The model under review builds one solid part; all positions refer to its coordinate system, in mm. Face numbers are marked on the shaded views. A direction names the side the tool comes from. Round coordinates to 2 decimals unless told otherwise and drop trailing zeros. Write each loop counter-clockwise with the first axis right and the second up, starting at its lowest first coordinate (ties: lowest second). Pieces come first, ordered by that corner, then holes. Notation, with made-up numbers: (60.5, 54) -> (89.5, 54) arc R19 ccw to (89.5, 64) -> close; hole circle Ø4 at (-28.5, 1.5). An arc over 180 degrees is marked (long way). Use CSV: the item, a comma, the result in double quotes. Start each with the question number.
1) Take a section at A-A, the plane x = 22.5. Give the boundary of the cut face in (y, z).
2) Machinability: for the marked faces 1, 2, 3 and 4, which of the approach directions +Z, -Z, +X, -X, +Y, -Y give a long, thin tool a straight path to every point of the face, cutting with its end or side? Answer none if there is none.
3) Take a section at C-C, the plane y = -6.75. Give the boundary of the cut face in (x, z).
4) Mouldability with a two-part tool opening along X and no side actions: class the marked faces 5, 6, 7 and 8 as released by +X, released by -X, zero draft, split by the parting line, or undercut.
5) Wall thickness on probe 1 along X at (y, z) = (9.75, 4.25); probe 2 along Y at (x, z) = (0, 8.25); probe 3 along Y at (x, z) = (4.5, 5.5): over which ranges is each line inside the solid? List them lowest first. Write a range as [from, to].
6) For pin 1 Ø8 at (x, y) = (27.5, 11.5) entering from +Z; pin 2 Ø3 at (y, z) = (8, 5.5) entering from +X; pin 3 Ø5 at (x, z) = (28, 3.5) entering from +Y; pin 4 Ø5 at (x, z) = (25, 7) entering from -Y, all flat-tipped, find the tip position at first contact; note any pin that passes through.
7) Take a section at B-B, the plane z = 2.5. State how many separate pieces and enclosed holes the cut face has, then the cut area to 3 significant figures.
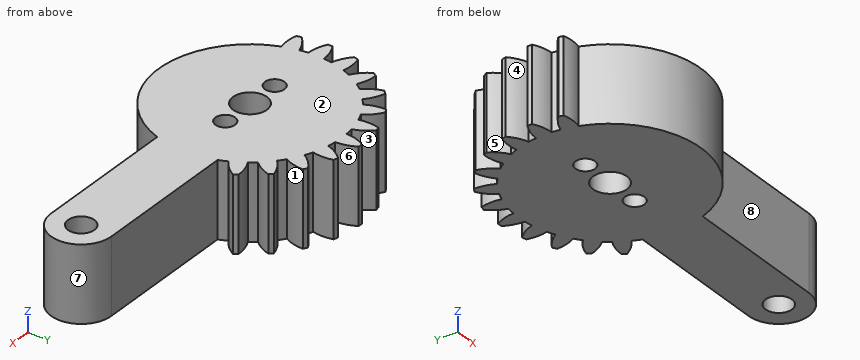
from build123d import *

# Parameters (mm, degrees)
SKETCH1_R           = 1.75
BOSS_EXTRUDE1_DEPTH = 10
SKETCH2_R           = 1.3
SKETCH2_R_2         = 2.25
CUT_EXTRUDE1_DEPTH  = 40.007683858


with BuildPart() as part:
    # Sketch1 → Boss-Extrude1 (new body)
    with BuildSketch(Plane.XY):
        with BuildLine():
            Line((0.31, 14.63), (-0.31, 14.63))
            ThreePointArc((-0.31, 14.63), (-0.838273314, 13.383704325), (-1.04, 12.04518576))
            ThreePointArc((-1.04, 12.04518576), (-1.578061664, 11.986568374), (-2.112960617, 11.903927815))
            ThreePointArc((-2.112960617, 11.903927815), (-2.65424773, 13.144626757), (-3.487085624, 14.211728743))
            Line((-3.487085624, 14.211728743), (-4.085959636, 14.051260935))
            ThreePointArc((-4.085959636, 14.051260935), (-4.273667417, 12.71070456), (-4.122086336, 11.365584201))
            ThreePointArc((-4.122086336, 11.365584201), (-4.626642697, 11.169703548), (-5.12192646, 10.951436862))
            ThreePointArc((-5.12192646, 10.951436862), (-5.965886177, 12.009764599), (-7.046532125, 12.824951657))
            Line((-7.046532125, 12.824951657), (-7.583467875, 12.514951657))
            ThreePointArc((-7.583467875, 12.514951657), (-7.417818147, 11.171491285), (-6.9232593, 9.911436862))
            ThreePointArc((-6.9232593, 9.911436862), (-7.359925677, 9.591641884), (-7.781841479, 9.252623584))
            ThreePointArc((-7.781841479, 9.252623584), (-8.870959341, 10.05645683), (-10.125769107, 10.564175311))
            Line((-10.125769107, 10.564175311), (-10.564175311, 10.125769107))
            ThreePointArc((-10.564175311, 10.125769107), (-10.05645683, 8.870959341), (-9.252623584, 7.781841479))
            ThreePointArc((-9.252623584, 7.781841479), (-9.591641884, 7.359925677), (-9.911436862, 6.9232593))
            ThreePointArc((-9.911436862, 6.9232593), (-11.171491285, 7.417818147), (-12.514951657, 7.583467875))
            Line((-12.514951657, 7.583467875), (-12.824951657, 7.046532125))
            ThreePointArc((-12.824951657, 7.046532125), (-12.009764599, 5.965886177), (-10.951436862, 5.12192646))
            ThreePointArc((-10.951436862, 5.12192646), (-11.169703548, 4.626642697), (-11.365584201, 4.122086336))
            ThreePointArc((-11.365584201, 4.122086336), (-12.71070456, 4.273667417), (-14.051260935, 4.085959636))
            Line((-14.051260935, 4.085959636), (-14.211728743, 3.487085624))
            ThreePointArc((-14.211728743, 3.487085624), (-13.144626757, 2.65424773), (-11.903927815, 2.112960617))
            ThreePointArc((-11.903927815, 2.112960617), (-11.986568374, 1.578061664), (-12.04518576, 1.04))
            ThreePointArc((-12.04518576, 1.04), (-13.383704325, 0.838273314), (-14.63, 0.31))
            Line((-14.63, 0.31), (-14.63, -0.31))
            ThreePointArc((-14.63, -0.31), (-13.383704325, -0.838273314), (-12.04518576, -1.04))
            ThreePointArc((-12.04518576, -1.04), (-11.986568374, -1.578061664), (-11.903927815, -2.112960617))
            ThreePointArc((-11.903927815, -2.112960617), (-13.144626757, -2.65424773), (-14.211728743, -3.487085624))
            Line((-14.211728743, -3.487085624), (-14.051260935, -4.085959636))
            ThreePointArc((-14.051260935, -4.085959636), (-12.71070456, -4.273667417), (-11.365584201, -4.122086336))
            ThreePointArc((-11.365584201, -4.122086336), (0.064808849, -12.089826294), (11.409123542, -4))
            Line((11.409123542, -4), (30.75, -4))
            ThreePointArc((30.75, -4), (34.75, 0), (30.75, 4))
            Line((30.75, 4), (11.409123542, 4))
            ThreePointArc((11.409123542, 4), (11.194344337, 4.566700654), (10.951436862, 5.12192646))
            ThreePointArc((10.951436862, 5.12192646), (12.009764599, 5.965886177), (12.824951657, 7.046532125))
            Line((12.824951657, 7.046532125), (12.514951657, 7.583467875))
            ThreePointArc((12.514951657, 7.583467875), (11.171491285, 7.417818147), (9.911436862, 6.9232593))
            ThreePointArc((9.911436862, 6.9232593), (9.591641884, 7.359925677), (9.252623584, 7.781841479))
            ThreePointArc((9.252623584, 7.781841479), (10.05645683, 8.870959341), (10.564175311, 10.125769107))
            Line((10.564175311, 10.125769107), (10.125769107, 10.564175311))
            ThreePointArc((10.125769107, 10.564175311), (8.870959341, 10.05645683), (7.781841479, 9.252623584))
            ThreePointArc((7.781841479, 9.252623584), (7.359925677, 9.591641884), (6.9232593, 9.911436862))
            ThreePointArc((6.9232593, 9.911436862), (7.417818147, 11.171491285), (7.583467875, 12.514951657))
            Line((7.583467875, 12.514951657), (7.046532125, 12.824951657))
            ThreePointArc((7.046532125, 12.824951657), (5.965886177, 12.009764599), (5.12192646, 10.951436862))
            ThreePointArc((5.12192646, 10.951436862), (4.626642697, 11.169703548), (4.122086336, 11.365584201))
            ThreePointArc((4.122086336, 11.365584201), (4.273667417, 12.71070456), (4.085959636, 14.051260935))
            Line((4.085959636, 14.051260935), (3.487085624, 14.211728743))
            ThreePointArc((3.487085624, 14.211728743), (2.65424773, 13.144626757), (2.112960617, 11.903927815))
            ThreePointArc((2.112960617, 11.903927815), (1.578061664, 11.986568374), (1.04, 12.04518576))
            ThreePointArc((1.04, 12.04518576), (0.838273314, 13.383704325), (0.31, 14.63))
        make_face()
        Circle(SKETCH1_R, mode=Mode.SUBTRACT)
        with Locations((30.75, 0)):
            Circle(SKETCH1_R, mode=Mode.SUBTRACT)
    extrude(amount=BOSS_EXTRUDE1_DEPTH)

    # Sketch2 → Cut-Extrude1 (cut, through all)
    with BuildSketch(Plane.XY.offset(10)):
        with Locations((-4.5, 0)):
            Circle(SKETCH2_R)
        with Locations((4.5, 0)):
            Circle(SKETCH2_R)
        Circle(SKETCH2_R_2)
    extrude(amount=-CUT_EXTRUDE1_DEPTH, mode=Mode.SUBTRACT)


solid = part.part
Values found:
1,outline,"(-4, 0) -> (4, 0) -> (4, 10) -> (-4, 10) -> close"
2,face 1,"+Z, -Z"
2,face 2,"+Z, +X, -X, +Y, -Y"
2,face 3,"+Z, -Z, +Y"
2,face 4,"+Z, -Z, -X"
3,outline,"(-10.03, 0) -> (10.03, 0) -> (10.03, 10) -> (-10.03, 10) -> close"
4,face 5,"released by -X"
4,face 6,"undercut"
4,face 7,"released by +X"
4,face 8,"zero draft"
5,probe 1,"[-10.45, -8.39], [-7.15, 7.15], [8.39, 10.45]"
5,probe 2,"[-12.09, -2.25], [2.25, 14.63]"
5,probe 3,"[-11.22, -1.3], [1.3, 11.22]"
6,pin 1,"through"
6,pin 2,"x = 12.82"
6,pin 3,"y = 4"
6,pin 4,"y = -4"
7,separate pieces,"1"
7,enclosed holes,"4"
7,area,"648 mm²"
